Design review of the part built by this model. Coordinates are the model's own, in mm. A direction names the side the tool comes from. Round coordinates to 2 decimals unless told otherwise and drop trailing zeros. Write each loop counter-clockwise with the first axis right and the second up, starting at its lowest first coordinate (ties: lowest second). Pieces come first, ordered by that corner, then holes. Notation, with made-up numbers: (56.25, 58.5) -> (102.25, 58.5) arc R24 cw to (102.25, 81.5) -> close; hole circle Ø1 at (49, -29.5). An arc over 180 degrees is marked (long way). Write item = value, one per line. Start each with the question number.
Item 1: Add section B-B, the plane z = -23.5. State the section outline as (x, y) points, then the cut area to 3 significant figures.
Item 2: Add section A-A, the plane y = -22. State the section outline as (x, z) points (3 decimals).
Item 3: To check wall thickness, follow L1, parallel to Z at x = -37.5, y = -7.5; L2, parallel to X at y = -14, z = 17.5; L3, parallel to X at y = -11, z = 46. State the ranges of each line that lie inside material, in increasing order.
Item 4: Machinability: for faces 5 (the flat face through (-27.963, -16, -4)), 6 (the flat face through (-47.013, -16, 45)), which of the approach directions +Z, -Z, +X, -X, +Y, -Y give a long, thin tool a straight path to every point of the face, cutting with its end or side? Answer none if there is none.
Item 5: For pin 1 Ø2 at (x, z) = (-54.5, -1.5) entering from +Y; pin 2 Ø7.5 at (x, y) = (-43, -14.5) entering from +Z; pin 3 Ø8 at (x, y) = (-60.5, -21.5) entering from -Z; pin 4 Ø9 at (y, z) = (-18, 39) entering from +X, all flat-tipped, find the tip position at first contact; note any pin that passes through.
Item 6: Mouldability with a two-part tool opening along Z and no side actions: class faces 1 (the cylindrical face through (-40.66, -15.65, 20.54)), 2 (the cylindrical face through (-29.41, -16.1, -30.52)), 3 (the cylindrical face through (-30.68, -16.1, 27.06)), 4 (the flat face through (-47.013, -16, -21)) as released by +Z, released by -Z, zero draft, split by the parting line, or undercut.
Item 7: Add section C-C, the plane x = -45. State the section outline as (y, z) points, then the cut area to 3 significant figures.
from build123d import *

# Parameters (mm, degrees)
F0_R     = 3.175
F1_DEPTH = 31.75
F2_R     = 5.08
F3_R     = 9.525


with BuildPart() as f1:
    # F0 (on Front) → F1 (new body)
    with BuildSketch(Plane.XZ):
        Polygon((-27.963307, 29.924871), (-47.013307, 29.924871), (-47.013307, 59.853119), (-66.063307, 59.853119), (-66.063307, 9.053119), (-47.013307, -9.996881), (-47.013307, -32.051129), (-27.963307, -32.051129), align=None)
        with Locations((-37.488307, 20.399871)):
            Circle(F0_R, mode=Mode.SUBTRACT)
    extrude(amount=F1_DEPTH)

    # F2
    f2_edges = [f1.edges().sort_by_distance(p)[0] for p in [
        (-27.963307, -15.875, -32.051129),
    ]]
    fillet(f2_edges, radius=F2_R)

    # F3
    f3_edges = [f1.edges().sort_by_distance(p)[0] for p in [
        (-27.963307, -15.875, 29.924871),
    ]]
    fillet(f3_edges, radius=F3_R)


solid = f1.part
Result set:
q1.outline = (-47.01, -31.75) -> (-27.96, -31.75) -> (-27.96, 0) -> (-47.01, 0) -> close
q1.area = 605 mm²
q2.outline = (-66.063, 9.053) -> (-47.013, -9.997) -> (-47.013, -32.051) -> (-33.043, -32.051) arc R5.08 ccw to (-27.963, -26.971) -> (-27.963, 20.4) arc R9.525 ccw to (-37.488, 29.925) -> (-47.013, 29.925) -> (-47.013, 59.853) -> (-66.063, 59.853) -> close; hole circle Ø6.35 at (-37.488, 20.4)
q3.L1 = -32.05 to 17.22, 23.57 to 29.92
q3.L2 = -66.06 to -38.78, -36.2 to -27.96
q3.L3 = -66.06 to -47.01
q4.face_5 = +Z, -Z, +X, +Y, -Y
q4.face_6 = +Z, +X, +Y, -Y
q5.pin_1 = 0
q5.pin_2 = 29.92
q5.pin_3 = -0.51
q5.pin_4 = -47.01
q6.face_1 = undercut
q6.face_2 = released by -Z
q6.face_3 = released by +Z
q6.face_4 = zero draft
q7.outline = (-31.75, -32.05) -> (0, -32.05) -> (0, 29.92) -> (-31.75, 29.92) -> close
q7.area = 1,970 mm²
